Could you check a few things on this model? Use its own coordinates, in mm. Coordinates: 2 decimals unless noted, no trailing zeros. Order: outer loops, then holes, each group sorted by start corner. A loop starts at its lowest first (then second) coordinate and runs counter-clockwise, first axis right, second up. Notation, with made-up numbers: (19.5, 82) - (52.5, 82) arc R34 ccw to (52.5, 118) - close; hole circle Ø10 at (-35.5, 20). An arc over 180 degrees is marked (long way). Answer as a JSON object with one key per item and string values. Group by question number.
(1) Imagine slicing it at B-B, the plane y = -32.5. Give the number of separate pieces and of enclosed holes in the cut face, and give its area (4 significant figures).
(2) Will this pin go through, and if not, where does the flat tip stop? P1, Ø20, axis at x = 62.5, y = -32.5, coming from the +Z side.
(3) Please list where these lines run through material, in increasing order: probe 1 along Y at (x, z) = (242.5, 0.85); probe 2 along Y at (x, z) = (18.5, 0.3); probe 3 along Y at (x, z) = (121, 0.4).
(4) We'd pull the mould along X, two halves only. Please class faces 1 (the cylindrical face through (24.22, -21.96, 0.99)), 2 (the cylindrical face through (119.423, -28.745, 0.993)), 3 (the flat face through (128, -32, 0)): pulls with the +X half, pulls with the -X half, needs draft (parallel to the pull), parting line crosses it, or undercut.
(5) Imagine slicing it at A-A, the plane x = 242.5. Write out the boundary of the cut face in (y, z), and give its area (3 significant figures).
from build123d import *

# Parameters (mm, degrees)
F0_W     = 260
F0_H     = 65
F0_R     = 12.5
F1_DEPTH = 2
F2_SIZE  = 0.5


with BuildPart() as f1:
    # F0 (on Top) → F1 (new body)
    with BuildSketch(Plane.XY):
        with Locations((130, -32.5)):
            Rectangle(F0_W, F0_H)
        with Locations((17.5, -32.5)):
            Circle(F0_R, mode=Mode.SUBTRACT)
        with Locations((62.5, -32.5)):
            Circle(F0_R, mode=Mode.SUBTRACT)
        with Locations((107.5, -32.5)):
            Circle(F0_R, mode=Mode.SUBTRACT)
        with Locations((152.5, -32.5)):
            Circle(F0_R, mode=Mode.SUBTRACT)
        with Locations((197.5, -32.5)):
            Circle(F0_R, mode=Mode.SUBTRACT)
        with Locations((242.5, -32.5)):
            Circle(F0_R, mode=Mode.SUBTRACT)
    extrude(amount=F1_DEPTH)

    # F2
    f2_edges = [f1.edges().sort_by_distance(p)[0] for p in [
        (130, 0, 2),
        (0, -32.5, 2),
        (130, -65, 2),
        (260, -32.5, 2),
        (5, -32.5, 2),
        (50, -32.5, 2),
        (95, -32.5, 2),
        (140, -32.5, 2),
        (185, -32.5, 2),
        (230, -32.5, 2),
        (130, 0, 0),
        (0, -32.5, 0),
        (130, -65, 0),
        (260, -32.5, 0),
        (5, -32.5, 0),
        (50, -32.5, 0),
        (95, -32.5, 0),
        (140, -32.5, 0),
        (185, -32.5, 0),
        (230, -32.5, 0),
    ]]
    chamfer(f2_edges, length=F2_SIZE)


solid = f1.part
Result set:
{
 "1": {"separate pieces": "7", "enclosed holes": "0", "area": "216.5 mm^2"},
 "2": {"P1": "passes through"},
 "3": {"probe 1": "y = -65 to -45, -20 to 0", "probe 2": "y = -64.8 to -45.16, -19.84 to -0.2", "probe 3": "y = -64.9 to -0.1"},
 "4": {"face 1": "undercut", "face 2": "undercut", "face 3": "needs draft"},
 "5": {"outline": "(-65, 0.5) - (-64.5, 0) - (-45.5, 0) - (-45, 0.5) - (-45, 1.5) - (-45.5, 2) - (-64.5, 2) - (-65, 1.5) - close; (-20, 0.5) - (-19.5, 0) - (-0.5, 0) - (0, 0.5) - (0, 1.5) - (-0.5, 2) - (-19.5, 2) - (-20, 1.5) - close", "area": "79.0 mm^2"}
}
